Geometry: final body of the model. Coordinates: model frame, mm. Round coordinates to 2 decimals unless told otherwise and drop trailing zeros. Loops run counter-clockwise (first coordinate to the right, second up) from the corner with the lowest first, then second, coordinate; pieces in that order, holes last. Notation, with made-up numbers: (39, 87.25) - (68, 87.25) arc R22 cw to (68, 112.25) - close; hole circle Ø3 at (65.25, 53). An arc over 180 degrees is marked (long way). Answer as CSV lines item,"result".
Autodesk Inventor part; units mm, degrees
ref_plane "YZ Plane" through (0, 0, 0) normal (1, 0, 0) x (0, 1, 0)
ref_plane "XZ Plane" through (0, 0, 0) normal (0, 1, 0) x (-1, 0, 0)
ref_plane "XY Plane" through (0, 0, 0) normal (0, 0, 1) x (1, 0, 0)
sketch "Sketch1" plane through (0, 0, 0) normal (0, 0, 1) x (1, 0, 0)
  line L0 (-23, 75) -> (23, 75)
  line L1 (25, 73) -> (25, -73)
  line L2 (23, -75) -> (-23, -75)
  line L3 (-25, -73) -> (-25, 73)
  arc A0 (-23, 75) -> (-25, 73) centre (-23, 73) ccw
  arc A1 (25, 73) -> (23, 75) centre (23, 73) ccw
  arc A2 (23, -75) -> (25, -73) centre (23, -73) ccw
  arc A3 (-25, -73) -> (-23, -75) centre (-23, -73) ccw
  point P0 (0, 0)
  point P1 (-25, 75)
  point P2 (25, 75)
  point P3 (-25, -75)
  point P4 (-25, 0)
  dimension "d0" = 50
  dimension "d1" = 150
  dimension "d2" = 25
  dimension "d3" = 75
  dimension "d4" = 2
  dimension "d5" = 2
  dimension "d6" = 2
  dimension "d7" = 2
extrude "Extrusion1" add sketch "Sketch1" along normal blind 2
sketch "Sketch2" plane through (0, 0, 2) normal (0, 0, 1) x (1, 0, 0)
  line L0 (-64, 0) -> (59, 0)
  line L1 (0, 89) -> (0, -64)
  line L2 (-25, 73) -> (-25, -73)
  line L3 (23, 75) -> (-23, 75)
  point P0 (0, 0)
  point P1 (-12.5, 50)
  point P2 (-12.5, 0)
  point P3 (-12.5, -50)
  point P4 (12.5, 50)
  point P5 (12.5, 0)
  point P6 (12.5, -50)
  dimension "d12" = 50
  dimension "d15" = 25
  dimension "d18" = 12.5
  dimension "d19" = 25
hole "Hole1" at (-12.5, 50, 2) at (-12.5, 0, 2) at (-12.5, -50, 2) at (12.5, 50, 2) at (12.5, 0, 2) at (12.5, -50, 2) direction (0, 0, -1) diameter 5 end through all
properties part number "joint"
(1) Section A-A (x = -12.5). Output: boundary loops of the cut face in (y, z).
Findings below:
outline,"(-75, 0) - (-52.5, 0) - (-52.5, 2) - (-75, 2) - close; (-47.5, 0) - (-2.5, 0) - (-2.5, 2) - (-47.5, 2) - close; (2.5, 0) - (47.5, 0) - (47.5, 2) - (2.5, 2) - close; (52.5, 0) - (75, 0) - (75, 2) - (52.5, 2) - close"
(2) Section B-B (z = 0.75). Output: boundary loops of the cut face in (x, y).
Findings below:
outline,"(-25, -73) arc R2 ccw to (-23, -75) - (23, -75) arc R2 ccw to (25, -73) - (25, 73) arc R2 ccw to (23, 75) - (-23, 75) arc R2 ccw to (-25, 73) - close; hole circle Ø5 at (-12.5, -50); hole circle Ø5 at (-12.5, 0); hole circle Ø5 at (-12.5, 50); hole circle Ø5 at (12.5, -50); hole circle Ø5 at (12.5, 0); hole circle Ø5 at (12.5, 50)"
(3) Section C-C (y = 50). Output: boundary loops of the cut face in (x, z).
Findings below:
outline,"(-25, 0) - (-15, 0) - (-15, 2) - (-25, 2) - close; (-10, 0) - (10, 0) - (10, 2) - (-10, 2) - close; (15, 0) - (25, 0) - (25, 2) - (15, 2) - close"
(4) Pin query (flat end, axial travel): P1, Ø6.5, axis at x = 12.5, y = 50, coming from the +Z side. Return the tip coordinate at first contact, or that it passes through.
Findings below:
P1,"z = 2"
(5) Material intervals for line 1 along Y through (x, z) = (12.5, 0.5); line 2 along X through (y, z) = (50, 0.55); line 3 along X through (y, z) = (48, 1.5), sorted ascending.
Findings below:
line 1,"-75 to -52.5, -47.5 to -2.5, 2.5 to 47.5, 52.5 to 75"
line 2,"-25 to -15, -10 to 10, 15 to 25"
line 3,"-25 to -14, -11 to 11, 14 to 25"
(6) Draft query along Y for faces 1 (the face through (-10.06, 0.54, 0.99)), 2 (the face through (0, 1, 0)), 3 (the face through (-10.28, -51.15, 0.99)). Return one class per face: pulls with the +Y half, pulls with the -Y half, needs draft (parallel to the pull), parting line crosses it, or undercut.
Findings below:
face 1,"undercut"
face 2,"needs draft"
face 3,"undercut"
